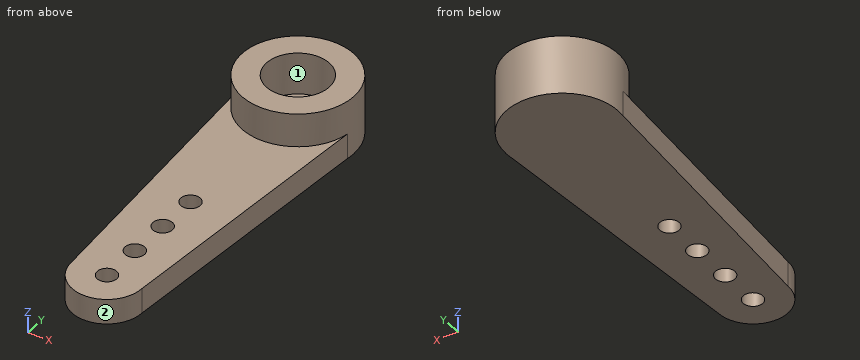
from build123d import *

# Parameters (mm, degrees)
ESBO_O1_R                = 4
ESBO_O1_R_2              = 2.25
RESSALTO_EXTRUS_O1_DEPTH = 4.2
ESBO_O3_R                = 0.7
RESSALTO_EXTRUS_O2_DEPTH = 1.8
ESBO_O4_R                = 2.5
RESSALTO_EXTRUS_O3_DEPTH = 1.2


with BuildPart() as part:
    # Esboço1 → Ressalto-extrusão1 (new body)
    with BuildSketch(Plane.XY):
        Circle(ESBO_O1_R)
        Circle(ESBO_O1_R_2, mode=Mode.SUBTRACT)
    extrude(amount=RESSALTO_EXTRUS_O1_DEPTH)

    # Esboço3 → Ressalto-extrusão2 (add)
    with BuildSketch(Plane.XY):
        with BuildLine():
            ThreePointArc((-2.5, -20.565998313), (0, -23.065998313), (2.5, -20.565998313))
            Line((2.5, -20.565998313), (3.957668004, -0.580399834))
            ThreePointArc((3.957668004, -0.580399834), (0, -4), (-3.957668004, -0.580399834))
            Line((-3.957668004, -0.580399834), (-2.5, -20.565998313))
        make_face()
        with Locations((0, -20.565998313)):
            Circle(ESBO_O3_R, mode=Mode.SUBTRACT)
        with Locations((0, -17.565998313)):
            Circle(ESBO_O3_R, mode=Mode.SUBTRACT)
        with Locations((0, -14.565998313)):
            Circle(ESBO_O3_R, mode=Mode.SUBTRACT)
        with Locations((0, -11.565998313)):
            Circle(ESBO_O3_R, mode=Mode.SUBTRACT)
    extrude(amount=RESSALTO_EXTRUS_O2_DEPTH)

    # Esboço4 → Ressalto-extrusão3 (add)
    with BuildSketch(Plane.XY):
        Circle(ESBO_O4_R)
    extrude(amount=RESSALTO_EXTRUS_O3_DEPTH)


solid = part.part
Input: part model. Units: mm. Frame: model coordinates. Face numbers are marked on the shaded views. A direction names the side the tool comes from. Give positions to 0.01 mm unless a question says otherwise; leave off trailing zeros. Order: outer loops, then holes, each group sorted by start corner. A loop starts at its lowest first (then second) coordinate and runs counter-clockwise, first axis right, second up. Notation, with made-up numbers: M -25.5,47.5 L -21.5,47.5 A7 ccw -21.5,59.5 Z; hole C 49,84 d3. An arc over 180 degrees is marked long. Answer as a JSON object with one key per item and string values.
1. First-contact query: P1, Ø1.3, axis at x = 0, y = -17.57, coming from the +Z side; P2, Ø2, axis at x = 2.5, y = -7.5, coming from the +Z side. Flat tips, straight axial feed; report the tip coordinate or a pass-through.
Result sheet:
{"P1": "through", "P2": "z = 1.8"}
2. Cut plane D-D, the plane x = -2. Output: boundary loops of the cut face in (y, z), and give its area (3 significant figures).
Result sheet:
{"outline": "M -22.07,0 L 3.46,0 L 3.46,4.2 L 1.03,4.2 L 1.03,1.2 L -1.03,1.2 L -1.03,4.2 L -3.46,4.2 L -3.46,1.8 L -22.07,1.8 Z", "area": "56.4 mm²"}
3. Cut plane C-C, the plane z = 3.35. Output: boundary loops of the cut face in (x, y).
Result sheet:
{"outline": "C 0,0 d8; hole C 0,0 d4.5"}
4. Cut plane B-B, the plane y = 0. Output: boundary loops of the cut face in (x, z).
Result sheet:
{"outline": "M -4,0 L 4,0 L 4,4.2 L 2.25,4.2 L 2.25,1.2 L -2.25,1.2 L -2.25,4.2 L -4,4.2 Z"}
5. Reachability of the marked faces 1 and 2 from +Z, -Z, +X, -X, +Y, -Y: full face, straight path, thin tool, end or side. Return the list, or none.
Result sheet:
{"face 1": "+Z", "face 2": "+Z, -Z, -Y"}
6. Cut plane A-A, the plane x = 0. Output: boundary loops of the cut face in (y, z).
Result sheet:
{"outline": "M -23.07,0 L -21.27,0 L -21.27,1.8 L -23.07,1.8 Z; M -19.87,0 L -18.27,0 L -18.27,1.8 L -19.87,1.8 Z; M -16.87,0 L -15.27,0 L -15.27,1.8 L -16.87,1.8 Z; M -13.87,0 L -12.27,0 L -12.27,1.8 L -13.87,1.8 Z; M -10.87,0 L 4,0 L 4,4.2 L 2.25,4.2 L 2.25,1.2 L -2.25,1.2 L -2.25,4.2 L -4,4.2 L -4,1.8 L -10.87,1.8 Z"}
7. Ray query, line 1 (Y direction, x = 0, z = 0.65); line 2 (Y direction, x = 0, z = 1.45); line 3 (Y direction, x = -0.5, z = 1.45). Return the intervals inside material, ascending. Write a range as [from, to].
Result sheet:
{"line 1": "[-23.07, -21.27], [-19.87, -18.27], [-16.87, -15.27], [-13.87, -12.27], [-10.87, 4]", "line 2": "[-23.07, -21.27], [-19.87, -18.27], [-16.87, -15.27], [-13.87, -12.27], [-10.87, -2.25], [2.25, 4]", "line 3": "[-23.02, -21.06], [-20.08, -18.06], [-17.08, -15.06], [-14.08, -12.06], [-11.08, -2.19], [2.19, 3.97]"}
